```python
from build123d import *

# Parameters (mm, degrees)
SKIZZE1_R                       = 1.59999934
AUFSATZ_LINEAR_AUSTRAGEN2_DEPTH = 1.6


with BuildPart() as part:
    # Skizze1 → Aufsatz-Linear austragen2 (new body)
    with BuildSketch(Plane(origin=(0, 0, 0), x_dir=(1, 0, 0), z_dir=(0, 1, 0))):
        with BuildLine():
            Line((0.000129244, 60.500005019), (-79.500003496, 60.499998316))
            ThreePointArc((-79.500003496, 60.499998316), (-83.389090307, 58.889085288), (-85.00000145, 54.999997696))
            Line((-85.00000145, 54.999997696), (-85.00000145, -54.999999283))
            ThreePointArc((-85.00000145, -54.999999283), (-83.389089945, -58.889083981), (-79.500005421, -60.499995903))
            Line((-79.500005421, -60.499995903), (-7.348e-06, -60.500004441))
            Line((-7.348e-06, -60.500004441), (79.499997674, -60.499997739))
            ThreePointArc((79.499997674, -60.499997739), (83.389083246, -58.889085422), (84.9999951, -54.999999659))
            Line((84.9999951, -54.999999659), (84.999993197, -0.063514366))
            ThreePointArc((84.999993197, -0.063514366), (84.936493195, -1.4365e-05), (84.999993199, 0.063485634))
            Line((84.999993199, 0.063485634), (84.99999637, 54.999998527))
            ThreePointArc((84.99999637, 54.999998527), (83.389084516, 58.889084164), (79.499999071, 60.499996481))
            Line((79.499999071, 60.499996481), (0.000129244, 60.500005019))
        make_face()
        with Locations(Location((-69.9999997, -54.00000122, 0), (0, 0, 270))):
            Circle(SKIZZE1_R, mode=Mode.SUBTRACT)
        with Locations(Location((69.9999997, -54.00000122, 0), (0, 0, 270))):
            Circle(SKIZZE1_R, mode=Mode.SUBTRACT)
        with Locations(Location((-69.9999997, 54.00000122, 0), (0, 0, 270))):
            Circle(SKIZZE1_R, mode=Mode.SUBTRACT)
        with Locations(Location((69.9999997, 54.00000122, 0), (0, 0, 270))):
            Circle(SKIZZE1_R, mode=Mode.SUBTRACT)
    extrude(amount=AUFSATZ_LINEAR_AUSTRAGEN2_DEPTH)


solid = part.part
```
Geometry check sheet. Reference: the model listing, model coordinates, mm. Coordinates: 2 decimals unless noted, no trailing zeros. Answer in a Markdown table with one row per item. Add a question column.
1. Gauge pin test, flat ends, axial feed: pin 1 Ø1 at (x, z) = (-22.5, 46.5) entering from -Y; pin 2 Ø2.5 at (x, z) = (-70, 54) entering from -Y. Record the tip position at first contact, or that the pin passes through.
2. Material ranges on L1, parallel to X at y = 1.55, z = 54.5; L2, parallel to X at y = 0.85, z = 53, recorded low to high. Write a range as [from, to].
3. Draft check along Z on faces 1 (the face through (83.43, 0.79, -58.85)), 2 (the face through (-83.43, 0.79, 58.85)), 3 (the face through (69.03, 0.79, 52.73)). Enter one of: +Z half, -Z half, draft (parallel to the pull), parting line (faces both ways), or undercut.
Data:
| question | item | result |
|---|---|---|
| 1 | pin 1 | stops at y = 0 |
| 1 | pin 2 | passes through |
| 2 | L1 | x = [-85, -71.52], [-68.48, 68.48], [71.52, 85] |
| 2 | L2 | x = [-85, -71.25], [-68.75, 68.75], [71.25, 85] |
| 3 | face 1 | -Z half |
| 3 | face 2 | +Z half |
| 3 | face 3 | undercut |
